Check sheet for the modelled part. Datum: model origin and axes. Units: mm. Face numbers are marked on the shaded views. Coordinates: 2 decimals unless noted, no trailing zeros. Order: outer loops, then holes, each group sorted by start corner. A loop starts at its lowest first (then second) coordinate and runs counter-clockwise, first axis right, second up. Notation, with made-up numbers: M 72,1 L 123,1 A10 ccw 123,13 Z; hole C -20,-13.75 d4. An arc over 180 degrees is marked long. Answer in a Markdown table with one row per item. Add a question column.
from build123d import *

# Parameters (mm, degrees)
SKETCH1_R           = 3
SKETCH2_R           = 7
SKETCH3_R           = 2
CUT_EXTRUDE1_DEPTH  = 8
FILLET1_R           = 0.45
FILLET2_R           = 0.4
SKETCH4_R           = 14.5
BOSS_EXTRUDE1_DEPTH = 1.8
SKETCH5_R           = 25
BOSS_EXTRUDE2_DEPTH = 3
FILLET3_R           = 3
SKETCH7_R           = 14.5
SKETCH6_R           = 22
SKETCH8_R           = 25
BOSS_EXTRUDE3_DEPTH = 7
FILLET4_R           = 7


with BuildPart() as part:
    # Sketch1 → Loft1 section 0
    with BuildSketch(Plane(origin=(0, 0, 0), x_dir=(1, 0, 0), z_dir=(0, 1, 0))):
        Circle(SKETCH1_R)
    # Sketch2 → Loft1 section 1
    with BuildSketch(Plane(origin=(0, 8, 0), x_dir=(1, 0, 0), z_dir=(0, 1, 0))):
        Circle(SKETCH2_R)
    loft()

    # Sketch3 → Cut-Extrude1 (cut)
    with BuildSketch(Plane.XZ):
        with Locations(Location((0, 0, 0), (0, 0, 270))):
            Circle(SKETCH3_R)
    extrude(amount=-CUT_EXTRUDE1_DEPTH, mode=Mode.SUBTRACT)

    # Fillet1
    fillet1_edges = [part.edges().sort_by_distance(p)[0] for p in [
        (-3, 0, 0),
    ]]
    fillet(fillet1_edges, radius=FILLET1_R)

    # Fillet2
    fillet2_edges = [part.edges().sort_by_distance(p)[0] for p in [
        (0, 0, 2),
    ]]
    fillet(fillet2_edges, radius=FILLET2_R)

    # Sketch4 → Boss-Extrude1 (add)
    with BuildSketch(Plane(origin=(0, 8, 0), x_dir=(1, 0, 0), z_dir=(0, 1, 0))):
        with Locations(Location((0, 0, 0), (0, 0, 270))):
            Circle(SKETCH4_R)
    extrude(amount=BOSS_EXTRUDE1_DEPTH)



with BuildPart() as body_2:
    # Sketch5 → Boss-Extrude2 (new body)
    with BuildSketch(Plane(origin=(0, 17.8, 0), x_dir=(1, 0, 0), z_dir=(0, 1, 0))):
        with Locations(Location((0, 0, 0), (0, 0, 270))):
            Circle(SKETCH5_R)
    extrude(amount=BOSS_EXTRUDE2_DEPTH)

    # Fillet3
    fillet3_edges = [body_2.edges().sort_by_distance(p)[0] for p in [
        (0, 17.8, -25),
    ]]
    fillet(fillet3_edges, radius=FILLET3_R - 0.0001)  # a hair under: the kernel refuses the full size


with BuildPart() as part_1:
    add(part.part)

    add(body_2.part)  # Loft3 merges body 2
    # Sketch7 → Loft3 section 0
    with BuildSketch(Plane(origin=(0, 9.8, 0), x_dir=(1, 0, 0), z_dir=(0, 1, 0))):
        Circle(SKETCH7_R)
    # Sketch6 → Loft3 section 1
    with BuildSketch(Plane.XZ.offset(-17.8)):
        Circle(SKETCH6_R)
    loft()

    # Sketch8 → Boss-Extrude3 (add)
    with BuildSketch(Plane(origin=(0, 20.8, 0), x_dir=(1, 0, 0), z_dir=(0, 1, 0))):
        with Locations(Location((0, 0, 0), (0, 0, 270))):
            Circle(SKETCH8_R)
    extrude(amount=BOSS_EXTRUDE3_DEPTH)

    # Fillet4
    fillet4_edges = [part_1.edges().sort_by_distance(p)[0] for p in [
        (0, 27.8, -25),
    ]]
    fillet(fillet4_edges, radius=FILLET4_R)


solid = part_1.part
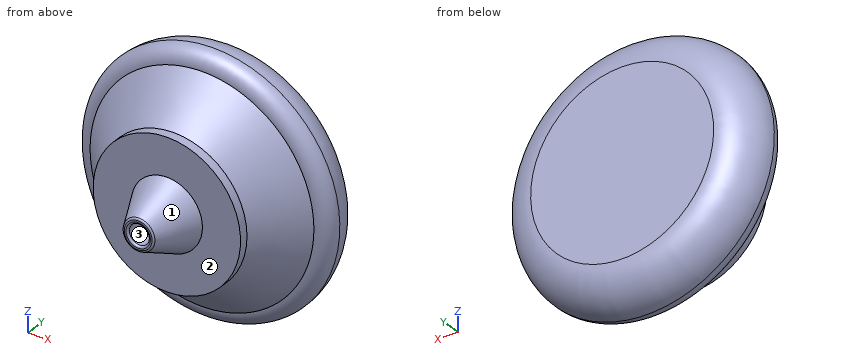
1. Section check B-B on y = 14. Enter the section's corners in (x, z) (1 decimal), then the cut area to 3 significant figures.
2. Go/stop test with flat-tipped pins: pin 1 Ø4.5 at (x, z) = (0.5, -1) entering from -Y; pin 2 Ø3 at (x, z) = (17.5, -7.5) entering from -Y; pin 3 Ø1.5 at (x, z) = (9, -15) entering from -Y; pin 4 Ø1.5 at (y, z) = (11, 7.5) entering from +X. Record where each tip stops, or that it passes through.
3. Release check for a two-part mould opening along Z. For the marked faces 1, 2 and 3 record: released by +Z, released by -Z, zero draft, split by the parting line, or undercut.
4. Scan lines: line 1 (Y direction, x = 8, z = 11.5); line 2 (X direction, y = 2, z = 0); line 3 (X direction, y = 2.5, z = 0). Record each from-to range of solid material in increasing order.
Result sheet:
| question | item | result |
|---|---|---|
| 1 | outline | C 0,0 d36.9 |
| 1 | area | 1,070 mm^2 |
| 2 | pin 1 | y = 0 |
| 2 | pin 2 | y = 13.04 |
| 2 | pin 3 | y = 12.19 |
| 2 | pin 4 | x = 14.59 |
| 3 | face 1 | split by the parting line |
| 3 | face 2 | zero draft |
| 3 | face 3 | undercut |
| 4 | line 1 | 8 to 27.8 |
| 4 | line 2 | -4 to -2, 2 to 4 |
| 4 | line 3 | -4.25 to -2, 2 to 4.25 |
